The listing builds one solid part. Answer for the finished solid, in the listing's coordinates (mm). Face numbers are marked on the shaded views. A direction names the side the tool comes from. Round coordinates to 2 decimals unless told otherwise and drop trailing zeros. Write each loop counter-clockwise with the first axis right and the second up, starting at its lowest first coordinate (ties: lowest second). Pieces come first, ordered by that corner, then holes. Notation, with made-up numbers: M 47.5,-10.75 L 80.5,-10.75 A32 cw 80.5,15.25 Z; hole C 80.5,76.5 d2. An arc over 180 degrees is marked long. Write each question's results on one line, items separated by ' | '.
from build123d import *

# Parameters (mm, degrees)
F0_W     = 105
F0_H     = 70
F1_DEPTH = 25
F2_R     = 12.5
F3_DEPTH = 7.5
F4_T     = -5
F6_W     = 95
F6_H     = 2.5
F7_DEPTH = 14.9
F8_W     = 2.5
F8_H     = 60
F9_DEPTH = 19.9
F10_R    = 5
F11_R    = 2


# Not quite as in the source:
# - an extrude ends at something that could not be found from the text; its depth is read off the source's solid


with BuildPart() as f1:
    # F0 (on Top) → F1 (new body)
    with BuildSketch(Plane.XY):
        with Locations((52.5, -35)):
            Rectangle(F0_W, F0_H)
    extrude(amount=F1_DEPTH)

    # F2 (on face) → F3 (join)
    with BuildSketch(Plane.XY.offset(25)):
        with Locations((17.5, -17.5)):
            Circle(F2_R)
        with Locations((52.5, -17.5)):
            Circle(F2_R)
        with Locations((87.5, -17.5)):
            Circle(F2_R)
        with Locations((17.5, -52.5)):
            Circle(F2_R)
        with Locations((52.5, -52.5)):
            Circle(F2_R)
        with Locations((87.5, -52.5)):
            Circle(F2_R)
    extrude(amount=F3_DEPTH)

    # F4
    f4_openings = [f1.faces().sort_by_distance(p)[0] for p in [
        (52.5, -35, 0),
    ]]
    offset(amount=F4_T, openings=f4_openings, kind=Kind.INTERSECTION)

    # F6 (on offset) → F7 (join, through all)
    with BuildSketch(Plane.XY.offset(5.1)):
        with Locations((52.5, -35)):
            Rectangle(F6_W, F6_H)
    extrude(amount=F7_DEPTH)

    # F8 (on offset) → F9 (join, through all)
    with BuildSketch(Plane.XY.offset(5.1)):
        with Locations((36.25, -35)):
            Rectangle(F8_W, F8_H)
        with Locations((68.75, -35)):
            Rectangle(F8_W, F8_H)
    extrude(amount=F9_DEPTH)

    # F10
    f10_edges = [f1.edges().sort_by_distance(p)[0] for p in [
        (5, -65, 10),
        (5, -5, 10),
        (100, -65, 10),
        (100, -5, 10),
    ]]
    fillet(f10_edges, radius=F10_R)

    # F11
    f11_edges = [f1.edges().sort_by_distance(p)[0] for p in [
        (105, -70, 12.5),
        (0, -70, 12.5),
        (0, 0, 12.5),
        (105, 0, 12.5),
    ]]
    fillet(f11_edges, radius=F11_R)


solid = f1.part
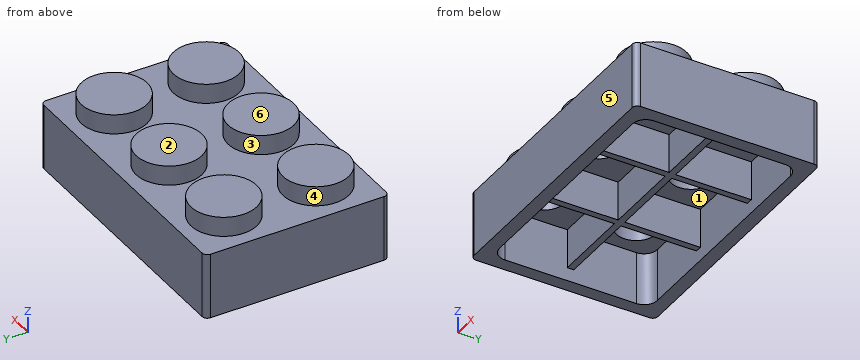
1) Section D-D (y = -42) is taken. Determine the outline of the cut face in (x, z).
Return value:
outline: M 0,0 L 5,0 L 5,20 L 35,20 L 35,5.1 L 37.5,5.1 L 37.5,20 L 67.5,20 L 67.5,5.1 L 70,5.1 L 70,20 L 100,20 L 100,0 L 105,0 L 105,25 L 94.28,25 L 94.28,32.5 L 80.72,32.5 L 80.72,25 L 59.28,25 L 59.28,32.5 L 45.72,32.5 L 45.72,25 L 24.28,25 L 24.28,32.5 L 10.72,32.5 L 10.72,25 L 0,25 Z
2) A tool of negligible diameter and unlimited length cuts with its end or side. For the marked faces 1, 2 and 3, from which of +Z, -Z, +X, -X, +Y, -Y can it reach the whole face along a straight path? Write none if from no direction.
Return value:
face 1: -Z | face 2: +Z, +X, -X, +Y, -Y | face 3: +Z
3) The mould has two halves that part along Y. Classify the marked faces 4, 5 and 6: +Y half, -Y half, draft (parallel to the pull), parting line (faces both ways), or undercut.
Return value:
face 4: undercut | face 5: -Y half | face 6: draft
4) Section A-A (z = 3.5) is taken. Determine the outline of the cut face in (x, y).
Return value:
outline: M 0,-68 A2 ccw 2,-70 L 103,-70 A2 ccw 105,-68 L 105,-2 A2 ccw 103,0 L 2,0 A2 ccw 0,-2 Z; hole M 5,-60 A5 ccw 10,-65 L 95,-65 A5 ccw 100,-60 L 100,-10 A5 ccw 95,-5 L 10,-5 A5 ccw 5,-10 Z
5) Section B-B (x = 52.5) is taken. Determine the outline of the cut face in (y, z).
Return value:
outline: M -70,0 L -65,0 L -65,20 L -60,20 L -60,27.5 L -45,27.5 L -45,20 L -36.25,20 L -36.25,5.1 L -33.75,5.1 L -33.75,20 L -25,20 L -25,27.5 L -10,27.5 L -10,20 L -5,20 L -5,0 L 0,0 L 0,25 L -5,25 L -5,32.5 L -30,32.5 L -30,25 L -40,25 L -40,32.5 L -65,32.5 L -65,25 L -70,25 Z
6) Section C-C (z = 30.5) is taken. Determine the outline of the cut face in (x, y).
Return value:
outline: C 17.5,-52.5 d25; C 17.5,-17.5 d25; C 52.5,-52.5 d25; C 52.5,-17.5 d25; C 87.5,-52.5 d25; C 87.5,-17.5 d25
7) Each of these flat-tipped pins is pushed along its axis until it touches: pin 1 (4 mm diameter, centred on x = 31.5, y = -39.5, fed in from +Z); pin 2 (12 mm diameter, centred on x = 21, y = -20.5, fed in from -Z); pin 3 (7.5 mm diameter, centred on x = 90.5, y = -19, fed in from -Z). Where does it stop, or does it pass through?
Return value:
pin 1: z = 25 | pin 2: z = 20 | pin 3: z = 27.5
8) Find the intervals of material crossed by line 1 (Y direction, x = 31.5, z = 12); line 2 (Y direction, x = 87.5, z = 23.5); line 3 (X direction, y = -52.5, z = 23.25), in increasing order.
Return value:
line 1: -70 to -65, -36.25 to -33.75, -5 to 0 | line 2: -70 to -60, -45 to -25, -10 to 0 | line 3: 0 to 10, 25 to 45, 60 to 80, 95 to 105
